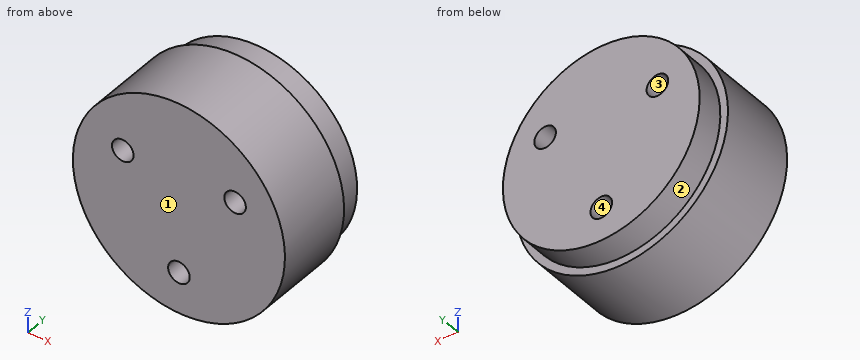
```python
from build123d import *

# Parameters (mm, degrees)
SKETCH2_R            = 27
BOSS_EXTRUDE2_DEPTH  = 27
M5_CLEARANCE_HOLE1_D = 5.5
CUT_EXTRUDE1_START   = -7
SKETCH10_R           = 27
SKETCH10_R_2         = 25.05
CUT_EXTRUDE1_DEPTH   = 7


with BuildPart() as part:
    # Sketch2 → Boss-Extrude2 (new body)
    with BuildSketch(Plane(origin=(0, 0, 0), x_dir=(1, 0, 0), z_dir=(0, 1, 0))):
        with Locations(Location((0, 0, 0), (0, 0, 270))):
            Circle(SKETCH2_R)
    extrude(amount=BOSS_EXTRUDE2_DEPTH)

    # M5 Clearance Hole1 (through all)
    with Locations(Plane(origin=(0, 0, 0), x_dir=(-1, 0, 0), z_dir=(0, -1, 0))):
        with Locations((14.298079416, -8.255), (0, 16.51), (-14.298079416, -8.255)):
            Hole(M5_CLEARANCE_HOLE1_D / 2)

    # Sketch10 → Cut-Extrude1 (cut)
    with BuildSketch(Plane(origin=(0, 27, 0), x_dir=(1, 0, 0), z_dir=(0, 1, 0)).offset(CUT_EXTRUDE1_START)):
        with Locations(Location((0, 0, 0), (0, 0, 270))):
            Circle(SKETCH10_R)
        with Locations(Location((0, 0, 0), (0, 0, 270))):
            Circle(SKETCH10_R_2, mode=Mode.SUBTRACT)
    extrude(amount=CUT_EXTRUDE1_DEPTH, mode=Mode.SUBTRACT)


solid = part.part
```
CAD build for the part. Positions are in the model's coordinates, mm. Face numbers are marked on the shaded views. Give positions to 0.01 mm unless a question says otherwise; leave off trailing zeros. Loops run counter-clockwise (first coordinate to the right, second up) from the corner with the lowest first, then second, coordinate; pieces in that order, holes last. Notation, with made-up numbers: M -0.5,86 L 22.5,86 A13 ccw 22.5,110 Z; hole C 31,45 d3. An arc over 180 degrees is marked long. Use one line per item in the form item = value.
Item 1: Slice it at B-B (z = -16.51). List the corners of the cut face in (x, y).
Determined:
outline = M -21.36,0 L -2.75,0 L -2.75,27 L -18.84,27 L -18.84,20 L -21.36,20 Z; M 2.75,0 L 21.36,0 L 21.36,20 L 18.84,20 L 18.84,27 L 2.75,27 Z
Item 2: Drill centre lines: probe 1 along Y at (x, z) = (25, 5); probe 2 along X at (y, z) = (16.75, -0.5); probe 3 along Z at (x, y) = (-14, 12.75). Where is each one in solid material? Low to high. Write a range as from..to.
Determined:
probe_1 = 0..20
probe_2 = -27..27
probe_3 = -23.09..5.52, 10.99..23.09
Item 3: Flat gauge pins, fed straight in: pin 1 (10 mm diameter, centred on x = -13.5, y = 16, fed in from +Z); pin 2 (8 mm diameter, centred on x = -19, y = 12.5, fed in from -Z); pin 3 (1.5 mm diameter, centred on y = 3, z = -20, fed in from +X). Where does each tip first touch, or does it go through?
Determined:
pin_1 = 25.63
pin_2 = -22.45
pin_3 = 18.93
Item 4: Slice it at A-A (x = 0). List the corners of the cut face in (y, z).
Determined:
outline = M 0,-27 L 20,-27 L 20,-25.05 L 27,-25.05 L 27,-19.26 L 0,-19.26 Z; M 0,-13.76 L 27,-13.76 L 27,25.05 L 20,25.05 L 20,27 L 0,27 Z
Item 5: Slice it at D-D (x = -19.5). List the corners of the cut face in (y, z), plus the area to 3 significant figures.
Determined:
outline = M 0,-18.67 L 20,-18.67 L 20,-15.72 L 27,-15.72 L 27,15.72 L 20,15.72 L 20,18.67 L 0,18.67 Z
area = 967 mm2
Item 6: Slice it at C-C (z = 0). List the corners of the cut face in (x, y), plus the area to 3 significant figures.
Determined:
outline = M -27,0 L 27,0 L 27,20 L 25.05,20 L 25.05,27 L -25.05,27 L -25.05,20 L -27,20 Z
area = 1,430 mm2
Item 7: Two-plate mould, pull along Z, no slides. Class the marked faces 1, 2, 3 and 4: pulls with the +Z half, pulls with the -Z half, needs draft (parallel to the pull), parting line crosses it, or undercut.
Determined:
face_1 = needs draft
face_2 = parting line crosses it
face_3 = undercut
face_4 = undercut
